Check sheet for the modelled part. Datum: model origin and axes. Units: mm. Round coordinates to 2 decimals unless told otherwise and drop trailing zeros. Order: outer loops, then holes, each group sorted by start corner. A loop starts at its lowest first (then second) coordinate and runs counter-clockwise, first axis right, second up.
Autodesk Fusion 360 part; units mm, degrees
sketch "Rectangle" plane through (0, 0, 0) normal (0, 0, 1) x (1, 0, 0)
  line L0 (45, -85) -> (-45, -85)
  line L1 (-45, -85) -> (-45, 85)
  line L2 (-45, 85) -> (45, 85)
  line L3 (45, 85) -> (45, -85)
  line L4 (45, -85) -> (-45, 85) construction
  line L5 (-45, -85) -> (45, 85) construction
extrude "Extrude1" add sketch "Rectangle" along normal blind 10
sketch "Diagonals" plane through (0, 0, 10) normal (0, 0, 1) x (-1, 0, 0)
  line L0 (-45, -85) -> (45, -85)
  line L1 (45, -85) -> (45, 85)
  line L2 (45, 85) -> (-45, 85)
  line L3 (-45, 85) -> (-45, -85)
  line L4 (45, -85) -> (-45, 85) construction
  line L5 (-45, -85) -> (45, 85) construction
  line L6 (45, -23.8236) -> (-45, 23.8235)
  dimension "d3" = 90
ref_plane "WorkPlane1" through (0, 0, 10) normal (0.8838, -0.4679, 0) x (0.4679, 0.8838, 0)
sketch "Circles" plane through (0, 0, 10) normal (0.8838, -0.4679, 0) x (0.4679, 0.8838, 0)
  circle A0 centre (0, 12) radius 5.831
  circle A1 centre (0, 12) radius 13.9284
extrude "Extrude2" add sketch "Circles" along normal mid plane 150
1) Draft check along Z on faces 1 (the face through (-1, 1, 0)), 2 (the face through (-1.5, -0.6, 27.7)), 3 (the face through (-1, 85, 5)). Enter one of: pulls with the +Z half, pulls with the -Z half, needs draft (parallel to the pull), parting line crosses it, or undercut.
2) Sectioned sample at B-B on y = -55.5. Record the cut outline in (x, z), and give its area (3 significant figures).
3) Scan lines: line 1 (X direction, y = -45, z = 7); line 2 (Z direction, x = 34.5, y = -1.5); line 3 (Z direction, x = -24, y = 4). Record each from-to range of solid material in increasing order.
4) Sectioned sample at C-C on z = 4.5. Record the cut outline in (x, y).
5) Gauge pin test, flat ends, axial feed: pin 1 (5 mm diameter, centred on x = -1, z = 11.5, fed in from +Y); pin 2 (2 mm diameter, centred on x = -28.5, y = -15.5, fed in from +Z); pin 3 (4 mm diameter, centred on y = -38, z = 6, fed in from +X); pin 4 (8 mm diameter, centred on y = 19, z = 31, fed in from +X). Record the tip position at first contact, or that the pin passes through.
6) Sectioned sample at A-A on z = 19.5. Record the cut outline in (x, y).
Values found:
1. face 1: pulls with the -Z half
1. face 2: undercut
1. face 3: needs draft
2. outline: (-45, 0) - (45, 0) - (45, 10) - (-45, 10) - close
2. area: 900 mm2
3. line 1: x = -45 to 45
3. line 2: z = 0 to 10
3. line 3: z = 0 to 10, 10.39 to 33.61
4. outline: (-45, -85) - (45, -85) - (45, 85) - (-45, 85) - close
5. pin 1: stops at y = 85
5. pin 2: stops at z = 10
5. pin 3: stops at x = 45
5. pin 4: stops at x = -3.6
6. outline: (-72.7, 22.98) - (59.87, -47.2) - (63.82, -39.75) - (-68.75, 30.44) - close; (-63.82, 39.75) - (68.75, -30.44) - (72.7, -22.98) - (-59.87, 47.2) - close
